Can you work these out from the model? Positions are in its coordinate system, mm. Face numbers are marked on the shaded views. A direction names the side the tool comes from. Round coordinates to 2 decimals unless told otherwise and drop trailing zeros. Loops run counter-clockwise (first coordinate to the right, second up) from the corner with the lowest first, then second, coordinate; pieces in that order, holes last. Notation, with made-up numbers: M 70,-15.75 L 118,-15.75 A17 cw 118,-10.75 Z; hole C -15,-31 d1. An arc over 180 degrees is marked long. Use a Markdown table: item, result. Add a question column.
```python
from build123d import *

# Parameters (mm, degrees)
SKETCH_1_R          = 24.5
SKETCH_1_R_2        = 1.5
EXTRUDE_1_DEPTH     = 5
SKETCH_2_R          = 2.5
EXTRUDE_2_DEPTH     = 5
SKETCH_4_R          = 1.25
CUT_EXTRUDE_1_DEPTH = 5
SKETCH_5_R          = 8
CUT_EXTRUDE_2_DEPTH = 5
SKETCH_6_R          = 2.5
CUT_EXTRUDE_3_DEPTH = 2


with BuildPart() as part:
    # 草图1 → 凸台-拉伸1 (new body)
    with BuildSketch(Plane.XY):
        Circle(SKETCH_1_R)
        with Locations((0, 12.5)):
            Circle(SKETCH_1_R_2, mode=Mode.SUBTRACT)
        with Locations((12.5, 0)):
            Circle(SKETCH_1_R_2, mode=Mode.SUBTRACT)
        with Locations((0, -12.5)):
            Circle(SKETCH_1_R_2, mode=Mode.SUBTRACT)
        with Locations((-12.5, 0)):
            Circle(SKETCH_1_R_2, mode=Mode.SUBTRACT)
    extrude(amount=EXTRUDE_1_DEPTH)

    # 草图2 → 凸台-拉伸2 (add)
    with BuildSketch(Plane.XY):
        with Locations((0, 19.25)):
            Circle(SKETCH_2_R)
        with Locations((19.25, 0)):
            Circle(SKETCH_2_R)
        with Locations((0, -19.25)):
            Circle(SKETCH_2_R)
        with Locations((-19.25, 0)):
            Circle(SKETCH_2_R)
    extrude(amount=-EXTRUDE_2_DEPTH)

    # 草图4 → 切除-拉伸1 (cut)
    with BuildSketch(Plane.XY):
        with Locations((0, 19.25)):
            Circle(SKETCH_4_R)
        with Locations((19.25, 0)):
            Circle(SKETCH_4_R)
        with Locations((0, -19.25)):
            Circle(SKETCH_4_R)
        with Locations((-19.25, 0)):
            Circle(SKETCH_4_R)
    extrude(amount=-CUT_EXTRUDE_1_DEPTH, mode=Mode.SUBTRACT)

    # 草图5 → 切除-拉伸2 (cut)
    with BuildSketch(Plane.XY):
        Circle(SKETCH_5_R)
    extrude(amount=CUT_EXTRUDE_2_DEPTH, mode=Mode.SUBTRACT)

    # 草图6 → 切除-拉伸3 (cut)
    with BuildSketch(Plane.XY):
        with Locations((0, 12.5)):
            Circle(SKETCH_6_R)
        with Locations((12.5, 0)):
            Circle(SKETCH_6_R)
        with Locations((0, -12.5)):
            Circle(SKETCH_6_R)
        with Locations((-12.5, 0)):
            Circle(SKETCH_6_R)
    extrude(amount=CUT_EXTRUDE_3_DEPTH, mode=Mode.SUBTRACT)


solid = part.part
```
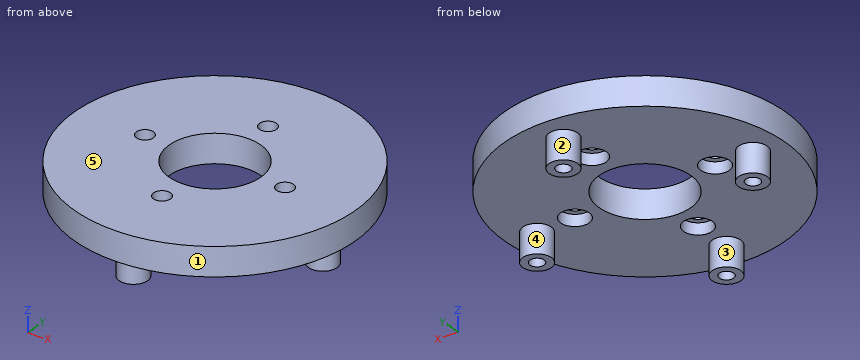
(1) If I drill on probe 1 along Y at (x, z) = (0, 1); probe 2 along Y at (x, z) = (0, 3.5); probe 3 along Z at (x, y) = (-4, -21.5), over which ranges is the centre line in solid material (lowest first)? Write a range as [from, to].
(2) On a 3-axis mill with a long thin cutter (end or side, diameter ignored), from which of +Z, -Z, +X, -X, +Y, -Y can I reach the whole of each face in a straight line? I mean the marked faces 1 and 2. Say none if no direction works.
(3) Suppose I cut it at A-A on z = -1. List the corners of the cut face in (x, y) for me.
(4) I'm going to push flat-ended pins straight in: pin 1 (1 mm diameter, centred on y = 19, z = 1.5, fed in from -X); pin 2 (1 mm diameter, centred on x = 3, z = 3, fed in from -Y); pin 3 (0.8 mm diameter, centred on x = 0, y = -19, fed in from -Z). Where does each tip first touch, or does it pass through?
(5) Suppose I cut it at C-C on z = 4. List the corners of the cut face in (x, y) for me, and give its area (3 significant figures).
(6) Suppose I cut it at B-B on y = 0. Count the separate pieces of the cut face and the enclosed holes in it, and give its area (3 significant figures).
(7) Suppose I cut it at D-D on x = -19.25. List the corners of the cut face in (y, z) for me.
(8) Thinking about a two-plate mould opening in Y: for the marked faces 3, 4 and 5, which applies, released by +Y, released by -Y, zero draft, split by the parting line, or undercut?
Results below:
| question | item | result |
|---|---|---|
| 1 | probe 1 | y = [-24.5, -15], [-10, -8], [8, 10], [15, 24.5] |
| 1 | probe 2 | y = [-24.5, -14], [-11, -8], [8, 11], [14, 24.5] |
| 1 | probe 3 | z = [0, 5] |
| 2 | face 1 | +Z, -Z |
| 2 | face 2 | -Z |
| 3 | outline | C -19.25,0 d5; C 0,-19.25 d5; C 0,19.25 d5; C 19.25,0 d5; hole C -19.25,0 d2.5; hole C 0,-19.25 d2.5; hole C 0,19.25 d2.5; hole C 19.25,0 d2.5 |
| 4 | pin 1 | stops at x = -16.06 |
| 4 | pin 2 | stops at y = -24.37 |
| 4 | pin 3 | stops at z = 0 |
| 5 | outline | C 0,0 d49; hole C -12.5,0 d3; hole C 0,0 d16; hole C 0,-12.5 d3; hole C 0,12.5 d3; hole C 12.5,0 d3 |
| 5 | area | 1,660 mm² |
| 6 | separate pieces | 4 |
| 6 | enclosed holes | 0 |
| 6 | area | 152 mm² |
| 7 | outline | M -15.16,0 L -2.5,0 L -2.5,-5 L -1.25,-5 L -1.25,0 L 1.25,0 L 1.25,-5 L 2.5,-5 L 2.5,0 L 15.16,0 L 15.16,5 L -15.16,5 Z |
| 8 | face 3 | undercut |
| 8 | face 4 | split by the parting line |
| 8 | face 5 | zero draft |
